For this review, use the dimensioned drawing (mm, ordinates from the lowest corner) and the shaded views. Round coordinates to 2 decimals unless told otherwise and drop trailing zeros. Loops run counter-clockwise (first coordinate to the right, second up) from the corner with the lowest first, then second, coordinate; pieces in that order, holes last. Notation, with made-up numbers: (34.5, 28) - (66.5, 28) arc R23 cw to (66.5, 51) - close; hole circle Ø4 at (-22.75, -38.5). An arc over 180 degrees is marked (long way). Use one line per item in the form item = value. Start each with the question number.
(1) We need section A-A, the plane x = 38.1. Write out the cut boundary in (y, z) (1 decimal).
(2) For pin 1 (6.5 mm diameter, centred on x = 38.1, y = 52.37, fed in from +Z); pin 2 (5.5 mm diameter, centred on x = 38.1, y = 26.52, fed in from +Z), all flat-tipped, find the tip position at first contact; note any pin that passes through.
(3) Wall thickness on probe 1 along Y at (x, z) = (38.1, 74) (1 decimal); probe 2 along X at (y, z) = (27, 35); probe 3 along Y at (x, z) = (38.1, 47) (1 decimal): over which ranges is each line inside the solid? List them lowest first. Write a range as [from, to].
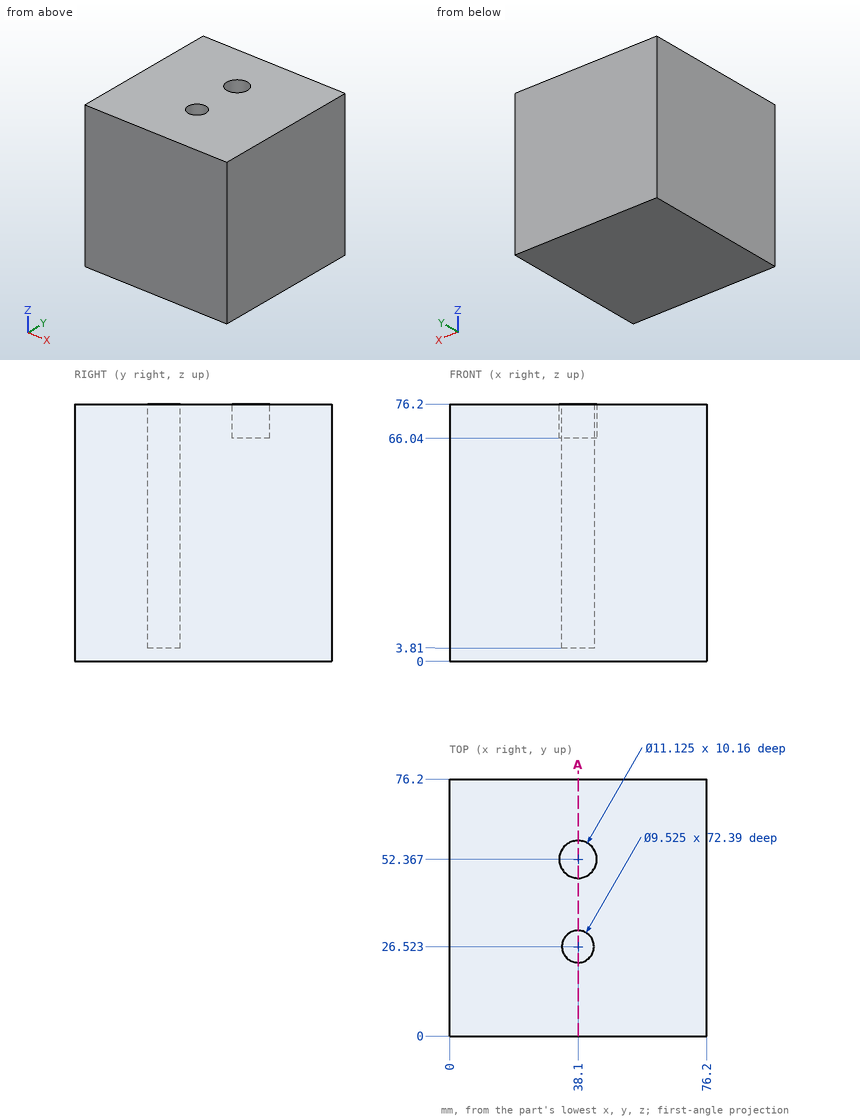
Data:
q1.outline = (0, 0) - (76.2, 0) - (76.2, 76.2) - (57.9, 76.2) - (57.9, 66) - (46.8, 66) - (46.8, 76.2) - (31.3, 76.2) - (31.3, 3.8) - (21.8, 3.8) - (21.8, 76.2) - (0, 76.2) - close
q2.pin_1 = 66.04
q2.pin_2 = 3.81
q3.probe_1 = [0, 21.8], [31.3, 46.8], [57.9, 76.2]
q3.probe_2 = [0, 33.36], [42.84, 76.2]
q3.probe_3 = [0, 21.8], [31.3, 76.2]
